For this review, take the finished solid that the model builds, in its own axes (mm). Face numbers are marked on the shaded views. A direction names the side the tool comes from. Coordinates: 2 decimals unless noted, no trailing zeros. Write each loop counter-clockwise with the first axis right and the second up, starting at its lowest first coordinate (ties: lowest second). Pieces come first, ordered by that corner, then holes. Notation, with made-up numbers: (-27, -38) -> (0, -38) arc R36 ccw to (0, 0) -> close; hole circle Ø6 at (5, 15). An arc over 180 degrees is marked (long way). Put each result on its own line as item: value. Start each with the question number.
Item 1: Consider section A-A on z = 40. Give the boundary of the cut face in (x, y), and give its area (3 significant figures).
Item 2: Consider section D-D on x = -8. Give the boundary of the cut face in (y, z).
Item 3: The part is to be moulded in two halves that separate along X. For the marked faces 5, 6, 7 and 8, say which applies: +X half, -X half, draft (parallel to the pull), parting line (faces both ways), or undercut.
Item 4: To check wall thickness, follow L1, parallel to Z at x = -4.5, y = 47.5; L2, parallel to X at y = 38.5, z = 36.5; L3, parallel to X at y = 45, z = 5.5. State the ranges of each line that lie inside material, in increasing order.
Item 5: For the marked faces 1, 2, 3 and 4, list the 3-axis set-ups (+Z, -Z, +X, -X, +Y, -Y) from which the entire face can be reached by the end or side of a thin tool; tool diameter is ignored.
Item 6: Consider section B-B on y = 50.5. Give the boundary of the cut face in (x, z).
Item 7: Insertion check: P1, Ø8.5, axis at x = 1, y = 46, coming from the -Z side; P2, Ø3, axis at x = -1, z = 21, coming from the +Y side; P3, Ø4, axis at y = 11.5, z = 8.5, coming from the +X side; P4, Ø1, axis at x = -22.5, z = 37.5, coming from the -Y side. Each pin has a flat end and moves straight along its axis. Give the tip position at first contact, or say it passes through.
Item 8: Consider section C-C on y = 35. Give the boundary of the cut face in (x, z), and give its area (3 significant figures).
```python
from build123d import *

# Parameters (mm, degrees)
BOSS_EXTRUDE1_DEPTH = 60
CUT_EXTRUDE1_START  = -52
SKETCH3_R           = 13.864092281
CUT_EXTRUDE1_DEPTH  = 44
SKETCH4_R           = 5
CUT_EXTRUDE2_DEPTH  = 90.75812925
SKETCH5_R           = 4.5
CUT_EXTRUDE3_DEPTH  = 15


with BuildPart() as part:
    # Sketch1 → Boss-Extrude1 (new body)
    with BuildSketch(Plane.XY):
        with BuildLine():
            Line((0, 0), (-35.793601182, 15.486061941))
            Line((-35.793601182, 15.486061941), (-35.793601182, 42.486061941))
            Line((-35.793601182, 42.486061941), (-14.301302797, 42.486061941))
            ThreePointArc((-14.301302797, 42.486061941), (-0.437210516, 56.350154222), (13.426881764, 42.486061941))
            Line((13.426881764, 42.486061941), (34.919180149, 42.486061941))
            Line((34.919180149, 42.486061941), (34.919180149, 21.486061941))
            Line((34.919180149, 21.486061941), (0, 0))
        make_face()
    extrude(amount=BOSS_EXTRUDE1_DEPTH)

    # Sketch3 → Cut-Extrude1 (cut)
    with BuildSketch(Plane.XY.offset(60).offset(CUT_EXTRUDE1_START)):
        with Locations((-0.437210516, 42.486061941)):
            Circle(SKETCH3_R)
    extrude(amount=CUT_EXTRUDE1_DEPTH, mode=Mode.SUBTRACT)

    # Sketch4 → Cut-Extrude2 (cut, through all)
    with BuildSketch(Plane.XY.offset(60)):
        with Locations((-0.437210516, 42.486061941)):
            Circle(SKETCH4_R)
    extrude(amount=-CUT_EXTRUDE2_DEPTH, mode=Mode.SUBTRACT)

    # Sketch5 → Cut-Extrude3 (cut)
    with BuildSketch(Plane(origin=(0, 0, 0), x_dir=(0.9177846456818411, -0.3970785113181741, 0), z_dir=(-0.3970785113181742, -0.9177846456818413, 0))):
        with Locations((-29, 51)):
            Circle(SKETCH5_R)
        with Locations((-29, 9)):
            Circle(SKETCH5_R)
    extrude(amount=-CUT_EXTRUDE3_DEPTH, mode=Mode.SUBTRACT)


solid = part.part
```
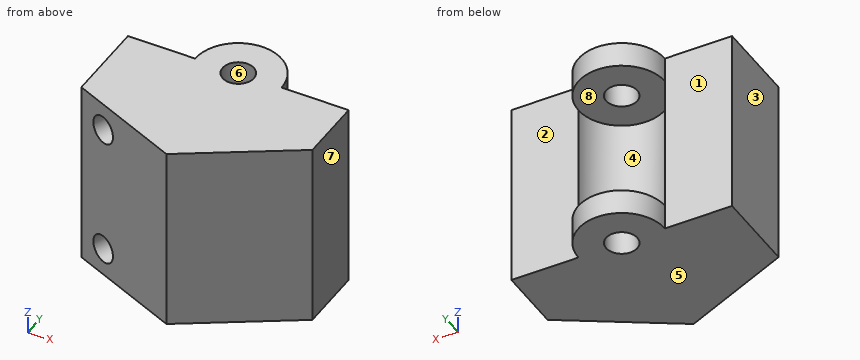
Return value:
1. outline: (-35.79, 15.49) -> (0, 0) -> (34.92, 21.49) -> (34.92, 42.49) -> (13.43, 42.49) arc R13.86 cw to (-14.3, 42.49) -> (-35.79, 42.49) -> close
1. area: 2,050 mm^2
2. outline: (3.46, 0) -> (54.11, 0) -> (54.11, 8) -> (30.87, 8) -> (30.87, 52) -> (54.11, 52) -> (54.11, 60) -> (3.46, 60) -> close
3. face 5: draft
3. face 6: undercut
3. face 7: +X half
3. face 8: undercut
4. L1: 0 to 8, 52 to 60
4. L2: -35.79 to -13.72, 12.84 to 34.92
4. L3: -14.07 to -4.76, 3.88 to 13.2
5. face 1: +Z, -Z, -X, +Y
5. face 2: +Z, -Z, +X, +Y
5. face 3: +Z, -Z, -X, +Y, -Y
5. face 4: +Y
6. outline: (-11.75, 0) -> (10.88, 0) -> (10.88, 8) -> (-11.75, 8) -> close; (-11.75, 52) -> (10.88, 52) -> (10.88, 60) -> (-11.75, 60) -> close
7. P1: z = 0
7. P2: y = 28.78
7. P3: x = 21.94
7. P4: y = 9.52
8. outline: (-35.79, 0) -> (34.92, 0) -> (34.92, 60) -> (-35.79, 60) -> close; hole (-12.11, 8) -> (11.23, 8) -> (11.23, 52) -> (-12.11, 52) -> close
8. area: 3,220 mm^2
